```python
from build123d import *

# Parameters (mm, degrees)
SKETCH1_W           = 60
SKETCH1_H           = 50
BOSS_EXTRUDE1_DEPTH = 40
SHELL1_T            = 2
SKETCH2_W           = 52
SKETCH2_H           = 40
CUT_EXTRUDE1_DEPTH  = 10
CHAMFER1_SIZE       = 4
SKETCH3_W           = 10
SKETCH3_H           = 10
CUT_EXTRUDE2_DEPTH  = 5
BOSS_EXTRUDE2_DEPTH = 6
CHAMFER3_SIZE       = 5
CHAMFER4_SIZE       = 4


with BuildPart() as part:
    # Sketch1 → Boss-Extrude1 (new body)
    with BuildSketch(Plane(origin=(0, 0, 0), x_dir=(1, 0, 0), z_dir=(0, 1, 0))):
        Rectangle(SKETCH1_W, SKETCH1_H)
    extrude(amount=BOSS_EXTRUDE1_DEPTH)

    # Shell1 (no face opened: a closed hollow body)
    add(offset(amount=-SHELL1_T, mode=Mode.PRIVATE), mode=Mode.SUBTRACT)

    # Sketch2 → Cut-Extrude1 (cut)
    with BuildSketch(Plane(origin=(0, 40, 0), x_dir=(1, 0, 0), z_dir=(0, 1, 0))):
        Rectangle(SKETCH2_W, SKETCH2_H)
    extrude(amount=-CUT_EXTRUDE1_DEPTH, mode=Mode.SUBTRACT)

    # Chamfer1
    chamfer1_edges = [part.edges().sort_by_distance(p)[0] for p in [
        (0, 0, 25),
        (-30, 0, 0),
        (0, 0, -25),
        (30, 0, 0),
    ]]
    chamfer(chamfer1_edges, length=CHAMFER1_SIZE)

    # Sketch3 → Cut-Extrude2 (cut)
    with BuildSketch(Plane(origin=(-30, 0, 0), x_dir=(0, 0, -1), z_dir=(1, 0, 0))):
        with Locations((0, 33)):
            Rectangle(SKETCH3_W, SKETCH3_H)
    extrude(amount=CUT_EXTRUDE2_DEPTH, mode=Mode.SUBTRACT)

    # Sketch4 → Boss-Extrude2 (add)
    with BuildSketch(Plane(origin=(-30, 0, 0), x_dir=(0, 0, -1), z_dir=(1, 0, 0))):
        Polygon((-5, 38), (-7, 38), (-7, 26), (7, 26), (7, 38), (5, 38), (5, 28), (-5, 28), align=None)
    extrude(amount=-BOSS_EXTRUDE2_DEPTH)

    # Chamfer3
    chamfer3_edges = [part.edges().sort_by_distance(p)[0] for p in [
        (-30, 26, 0),
    ]]
    chamfer(chamfer3_edges, length=CHAMFER3_SIZE)

    # Chamfer4
    chamfer4_edges = [part.edges().sort_by_distance(p)[0] for p in [
        (-32, 28, 5),
        (-32, 28, -5),
    ]]
    chamfer(chamfer4_edges, length=CHAMFER4_SIZE)


solid = part.part
```
Read the model definition and answer for the solid it produces. Units are mm, in the model's axes. A direction names the side the tool comes from. Coordinates: 2 decimals unless noted, no trailing zeros. Loops run counter-clockwise (first coordinate to the right, second up) from the corner with the lowest first, then second, coordinate; pieces in that order, holes last.
(1) Consider line 1 along X through (y, z) = (20.5, -11.5); line 2 along Z through (x, y) = (-12.5, 23); line 3 along Y through (x, z) = (-27, 16). Determine where each line is inside the solid, lowest interval first.
Solution:
line 1: x = -30 to -28, 28 to 30
line 2: z = -25 to -23, 23 to 25
line 3: y = 1 to 2, 38 to 40
(2) The part is cut by section D-D (y = 30). Determine the outline of the cut face in (x, z).
Solution:
outline: (-36, -7) - (-30, -7) - (-30, -25) - (30, -25) - (30, 25) - (-30, 25) - (-30, 7) - (-36, 7) - (-36, 3) - (-28, 3) - (-28, 23) - (28, 23) - (28, -23) - (-28, -23) - (-28, -3) - (-36, -3) - close
(3) Flat-ended cylindrical pins translate along their axes: pin 1 Ø0.6 at (y, z) = (39.5, -5) entering from -X; pin 2 Ø5 at (x, z) = (-16, -16) entering from +Y; pin 3 Ø1 at (x, z) = (-34, 5.5) entering from +Y. Find the tip coordinate at first contact, or state that the pin passes through.
Solution:
pin 1: stops at x = -30
pin 2: stops at y = 2
pin 3: stops at y = 38
(4) The part is cut by section C-C (y = 25). Determine the outline of the cut face in (x, z), and give its area (3 significant figures).
Solution:
outline: (-34, -7) - (-30, -7) - (-30, -25) - (30, -25) - (30, 25) - (-30, 25) - (-30, 7) - (-34, 7) - close; hole (-28, -23) - (28, -23) - (28, 23) - (-28, 23) - close
area: 480 mm2
(5) The mould has two halves that part along Y. Classify faces 6 (the face through (28, 20, 0)), 7 (the face through (-28.4, 2.4, 0.3)), 8 (the face through (-33, 38, 6)): released by +Y, released by -Y, zero draft, split by the parting line, or undercut.
Solution:
face 6: undercut
face 7: released by -Y
face 8: released by +Y
(6) A tool of negligible diameter and unlimited length cuts with its end or side. For faces 1 (the face through (-26, 39, 0)), 2 (the face through (-33, 32, 7)), 3 (the face through (-32, 35, -5)), 4 (the face through (0, 2, 0)), 5 (the face through (-33, 31, -7)), from which of +Z, -Z, +X, -X, +Y, -Y can it reach the whole face along a straight path? Write none if from no direction.
Solution:
face 1: +Y
face 2: +Z, -X, +Y, -Y
face 3: -X
face 4: none
face 5: -Z, -X, +Y, -Y
